The listing builds one solid part. Answer for the finished solid, in the listing's coordinates (mm). Face numbers are marked on the shaded views. Give positions to 0.01 mm unless a question says otherwise; leave off trailing zeros. Answer in a Markdown table with one row per item.
from build123d import *

# Parameters (mm, degrees)
SKETCH2_W          = 1.2
SKETCH2_H          = 12.675438596
CHAMFER2_SIZE      = 0.4
FILLET1_R          = 0.3
CUT_EXTRUDE2_DEPTH = 0.6
FILLET2_R          = 0.3


with BuildPart() as part:
    # Sketch2 → Revolve1 (revolve)
    with BuildSketch(Plane.XY, mode=Mode.PRIVATE) as revolve1_sk:
        with Locations((-5.85, 11.162280702)):
            Rectangle(SKETCH2_W, SKETCH2_H)
    revolve(revolve1_sk.sketch.rotate(Axis((0, 0, 0), (1, 0, 0)), 90), axis=Axis((0, 0, 0), (1, 0, 0)))

    # Sketch4 → Revolve2 (revolve)
    with BuildSketch(Plane.XY, mode=Mode.PRIVATE) as revolve2_sk:
        with BuildLine():
            Line((-5.25, 6.074561404), (-5.25, 4.824561404))
            Line((-5.25, 4.824561404), (3.8, 4.824561404))
            Line((3.8, 4.824561404), (3.8, 6.074561404))
            Line((3.8, 6.074561404), (-3.316987298, 6.074561404))
            ThreePointArc((-3.316987298, 6.074561404), (-3.75, 6.324561404), (-4.183012702, 6.074561404))
            Line((-4.183012702, 6.074561404), (-5.25, 6.074561404))
        make_face()
    revolve(revolve2_sk.sketch.rotate(Axis((0, 0, 0), (1, 0, 0)), 90), axis=Axis((0, 0, 0), (1, 0, 0)))

    # Chamfer2
    chamfer2_edges = [part.edges().sort_by_distance(p)[0] for p in [
        (3.8, 0, -6.074561404),
    ]]
    chamfer(chamfer2_edges, length=CHAMFER2_SIZE)

    # Fillet1
    fillet1_edges = [part.edges().sort_by_distance(p)[0] for p in [
        (-6.45, 0, -17.5),
        (-5.25, 0, -17.5),
    ]]
    fillet(fillet1_edges, radius=FILLET1_R)

    # Sketch3_3 → Cut-Extrude2 (cut)
    with BuildSketch(Plane.ZY.offset(6.45)):
        with BuildLine():
            Line((4.517828644, 5.048158729), (3.667716206, 4.198046292))
            ThreePointArc((3.667716206, 4.198046292), (2.133292292, 5.150223183), (0.375, 5.561934002))
            Line((0.375, 5.561934002), (0.375, 6.76417454))
            ThreePointArc((0.375, 6.76417454), (2.592512411, 6.258878622), (4.517828644, 5.048158729))
        make_face()
        with BuildLine():
            ThreePointArc((5.561934002, 0.375), (5.150223183, 2.133292292), (4.198046292, 3.667716206))
            Line((4.198046292, 3.667716206), (5.048158729, 4.517828644))
            ThreePointArc((5.048158729, 4.517828644), (6.258878622, 2.592512411), (6.76417454, 0.375))
            Line((6.76417454, 0.375), (5.561934002, 0.375))
        make_face()
        with BuildLine():
            ThreePointArc((0.375, -5.561934002), (2.133292292, -5.150223183), (3.667716206, -4.198046292))
            Line((3.667716206, -4.198046292), (4.517828644, -5.048158729))
            ThreePointArc((4.517828644, -5.048158729), (2.592512411, -6.258878622), (0.375, -6.76417454))
            Line((0.375, -6.76417454), (0.375, -5.561934002))
        make_face()
        with BuildLine():
            ThreePointArc((-3.667716206, -4.198046292), (-2.133292292, -5.150223183), (-0.375, -5.561934002))
            Line((-0.375, -5.561934002), (-0.375, -6.76417454))
            ThreePointArc((-0.375, -6.76417454), (-2.592512411, -6.258878622), (-4.517828644, -5.048158729))
            Line((-4.517828644, -5.048158729), (-3.667716206, -4.198046292))
        make_face()
        with BuildLine():
            ThreePointArc((-5.561934002, -0.375), (-5.150223183, -2.133292292), (-4.198046292, -3.667716206))
            Line((-4.198046292, -3.667716206), (-5.048158729, -4.517828644))
            ThreePointArc((-5.048158729, -4.517828644), (-6.258878622, -2.592512411), (-6.76417454, -0.375))
            Line((-6.76417454, -0.375), (-5.561934002, -0.375))
        make_face()
        with BuildLine():
            ThreePointArc((-4.198046292, 3.667716206), (-5.150223183, 2.133292292), (-5.561934002, 0.375))
            Line((-5.561934002, 0.375), (-6.76417454, 0.375))
            ThreePointArc((-6.76417454, 0.375), (-6.258878622, 2.592512411), (-5.048158729, 4.517828644))
            Line((-5.048158729, 4.517828644), (-4.198046292, 3.667716206))
        make_face()
        with BuildLine():
            ThreePointArc((-0.375, 5.561934002), (-2.133292292, 5.150223183), (-3.667716206, 4.198046292))
            Line((-3.667716206, 4.198046292), (-4.517828644, 5.048158729))
            ThreePointArc((-4.517828644, 5.048158729), (-2.592512411, 6.258878622), (-0.375, 6.76417454))
            Line((-0.375, 6.76417454), (-0.375, 5.561934002))
        make_face()
        with BuildLine():
            ThreePointArc((4.198046292, -3.667716206), (5.150223183, -2.133292292), (5.561934002, -0.375))
            Line((5.561934002, -0.375), (6.76417454, -0.375))
            ThreePointArc((6.76417454, -0.375), (6.258878622, -2.592512411), (5.048158729, -4.517828644))
            Line((5.048158729, -4.517828644), (4.198046292, -3.667716206))
        make_face()
    extrude(amount=-CUT_EXTRUDE2_DEPTH, mode=Mode.SUBTRACT)

    # Fillet2
    fillet2_edges = [part.edges().sort_by_distance(p)[0] for p in [
        (-6.15, 0.375, 5.561934002),
        (-6.15, 3.667716206, 4.198046292),
        (-6.15, 4.517828644, 5.048158729),
        (-6.15, 0.375, 6.76417454),
        (-6.15, -5.561934002, 0.375),
        (-6.15, -4.198046292, 3.667716206),
        (-6.15, -5.048158729, 4.517828644),
        (-6.15, -6.76417454, 0.375),
        (-6.15, -0.375, -5.561934002),
        (-6.15, -3.667716206, -4.198046292),
        (-6.15, -4.517828644, -5.048158729),
        (-6.15, -0.375, -6.76417454),
        (-6.15, -4.198046292, -3.667716206),
        (-6.15, -5.561934002, -0.375),
        (-6.15, -6.76417454, -0.375),
        (-6.15, -5.048158729, -4.517828644),
        (-6.15, 5.561934002, -0.375),
        (-6.15, 4.198046292, -3.667716206),
        (-6.15, 5.048158729, -4.517828644),
        (-6.15, 6.76417454, -0.375),
        (-6.15, 3.667716206, -4.198046292),
        (-6.15, 0.375, -5.561934002),
        (-6.15, 0.375, -6.76417454),
        (-6.15, 4.517828644, -5.048158729),
        (-6.15, -3.667716206, 4.198046292),
        (-6.15, -0.375, 5.561934002),
        (-6.15, -0.375, 6.76417454),
        (-6.15, -4.517828644, 5.048158729),
        (-6.15, 5.048158729, 4.517828644),
        (-6.15, 4.198046292, 3.667716206),
        (-6.15, 5.561934002, 0.375),
        (-6.15, 6.76417454, 0.375),
    ]]
    fillet(fillet2_edges, radius=FILLET2_R)


solid = part.part
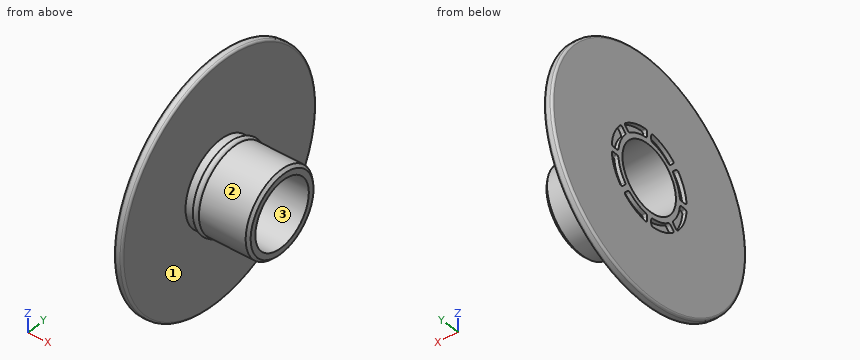
Item 1: Determine the mould class of the marked faces 1, 2 and 3 for opening direction Y: pulls with the +Y half, pulls with the -Y half, needs draft (parallel to the pull), parting line crosses it, or undercut.
Answer block:
| item | result |
|---|---|
| face 1 | needs draft |
| face 2 | parting line crosses it |
| face 3 | undercut |
Item 2: Each of these flat-tipped pins is pushed along its axis until it touches: P1, Ø5, axis at x = 0.5, z = -4, coming from the +Y side; P2, Ø3, axis at x = -4, y = 3.5, coming from the -Z side; P3, Ø0.7, axis at x = -6, y = -6, coming from the -Z side; P4, Ø6, axis at x = -1, y = -10, coming from the +Z side. Where does it stop, or does it pass through?
Answer block:
| item | result |
|---|---|
| P1 | y = 5.89 |
| P2 | z = -17.21 |
| P3 | z = -16.56 |
| P4 | through |
Item 3: Consider line 1 (Y direction, x = -3.25, z = 0); line 2 (Y direction, x = -3.75, z = 0); line 3 (X direction, y = -13, z = 2.5). Determine where each line is inside the solid, lowest interval first.
Answer block:
| item | result |
|---|---|
| line 1 | -6.07 to -4.82, 4.82 to 6.07 |
| line 2 | -6.32 to -4.82, 4.82 to 6.32 |
| line 3 | -6.45 to -5.25 |
